from build123d import *

# Parameters (mm, degrees)
SKETCH1_W                        = 330
SKETCH1_H                        = 43.5
BOSS_EXTRUDE1_DEPTH              = 8
SKETCH6_W                        = 25.004721381
SKETCH6_H                        = 24.5
SKETCH6_W_2                      = 25.004721382
CUT_EXTRUDE1_DEPTH               = 1
TAPPED_HOLE_FOR_4_40_HELICOIL2_D = 3.048


with BuildPart() as part:
    # Sketch1 → Boss-Extrude1 (new body)
    with BuildSketch(Plane(origin=(0, 0, 0), x_dir=(1, 0, 0), z_dir=(0, 1, 0))):
        with Locations((-165, 21.75)):
            Rectangle(SKETCH1_W, SKETCH1_H)
    extrude(amount=BOSS_EXTRUDE1_DEPTH)

    # Sketch6 → Cut-Extrude1 (cut)
    with BuildSketch(Plane(origin=(0, 8, 0), x_dir=(1, 0, 0), z_dir=(0, 1, 0))):
        with Locations((-213.007082072, 21.75)):
            Rectangle(SKETCH6_W, SKETCH6_H)
        with Locations((-181.002360691, 21.75)):
            Rectangle(SKETCH6_W_2, SKETCH6_H)
        with Locations((-245.011803454, 21.75)):
            Rectangle(SKETCH6_W_2, SKETCH6_H)
        with Locations((-277.016524836, 21.75)):
            Rectangle(SKETCH6_W_2, SKETCH6_H)
        with Locations((-309.021246217, 21.209761144)):
            Rectangle(SKETCH6_W, SKETCH6_H)
        with Locations((-148.997639309, 21.75)):
            Rectangle(SKETCH6_W_2, SKETCH6_H)
        with Locations((-116.992917928, 21.75)):
            Rectangle(SKETCH6_W, SKETCH6_H)
        with Locations((-84.988196546, 21.75)):
            Rectangle(SKETCH6_W_2, SKETCH6_H)
        with Locations((-52.983475164, 21.75)):
            Rectangle(SKETCH6_W_2, SKETCH6_H)
        with Locations((-20.978753783, 21.209761144)):
            Rectangle(SKETCH6_W, SKETCH6_H)
    extrude(amount=-CUT_EXTRUDE1_DEPTH, mode=Mode.SUBTRACT)

    # Tapped Hole for #4-40 Helicoil2 (through all)
    with Locations(Plane(origin=(0, 8, 0), x_dir=(1, 0, 0), z_dir=(0, 1, 0))):
        with Locations((-165, 39.745256998), (-165, 4.663980245), (-250, 4.663980245), (-325, 4.75), (-325, 38.75), (-250, 39.745256998), (-80, 39.745256998), (-80, 4.663980245), (-5, 4.663980245), (-5, 39.745256998)):
            Hole(TAPPED_HOLE_FOR_4_40_HELICOIL2_D / 2)


solid = part.part
CAD build for the part. Positions are in the model's coordinates, mm. A direction names the side the tool comes from. Round coordinates to 2 decimals unless told otherwise and drop trailing zeros. Loops run counter-clockwise (first coordinate to the right, second up) from the corner with the lowest first, then second, coordinate; pieces in that order, holes last.
(1) Cut at A-A (x = -111.5). Give the cut face in (y, z), plus the area to 4 significant figures.
(2) Drop a flat-ended pin along its axis: pin 1 (12 mm diameter, centred on x = -182, z = -19, fed in from +Y). Give the stop position or say it passes through.
(3) Wall check: line 1 along Z through (x, y) = (-165, 2.75); line 2 along X through (y, z) = (3.75, -6); line 3 along X through (y, z) = (6.75, -4.75). Give the ranges that are in metal, low to high.
(4) Which spindle directions (+Z, -Z, +X, -X, +Y, -Y) get a long thin tool onto all of the face, cutting with end or side? Do faces 1 (the flat face through (-213, 7, -22)), 2 (the flat face through (-167, 4, 0)). Say none if no direction does.
Findings below:
1. outline: (0, -43.5) - (8, -43.5) - (8, -34) - (7, -34) - (7, -9.5) - (8, -9.5) - (8, 0) - (0, 0) - close
1. area: 323.5 mm2
2. pin 1: stops at y = 7
3. line 1: z = -43.5 to -41.27, -38.22 to -6.19, -3.14 to 0
3. line 2: x = -330 to -325.87, -324.13 to -250.73, -249.27 to -165.73, -164.27 to -80.73, -79.27 to -5.73, -4.27 to 0
3. line 3: x = -330 to -326.52, -323.48 to -251.52, -248.48 to -166.52, -163.48 to -81.52, -78.48 to -6.52, -3.48 to 0
4. face 1: +Y
4. face 2: +Z, +X, -X, +Y, -Y
